```python
from build123d import *

# Parameters (mm, degrees)
SKETCH6_R               = 10
BOSS_EXTRUDE4_DEPTH     = 2.5
SKETCH7_R               = 6
BOSS_EXTRUDE5_DEPTH     = 6.4
SKETCH8_R               = 6
BOSS_EXTRUDE6_DEPTH     = 6.4
CUT_EXTRUDE1_DEPTH      = 7.4
CUT_EXTRUDE1_DEPTH_BACK = 12.4
FILLET1_R               = 0.5


with BuildPart() as part:
    # Sketch6 → Boss-Extrude4 (new body, symmetric)
    with BuildSketch(Plane.XY):
        Circle(SKETCH6_R)
    extrude(amount=BOSS_EXTRUDE4_DEPTH, both=True)

    # Sketch7 → Boss-Extrude5 (add)
    with BuildSketch(Plane.XY.offset(2.5)):
        with Locations((0, 1)):
            Circle(SKETCH7_R)
    extrude(amount=BOSS_EXTRUDE5_DEPTH)

    # Sketch8 → Boss-Extrude6 (add)
    with BuildSketch(Plane(origin=(0, 0, -2.5), x_dir=(-1, 0, 0), z_dir=(0, 0, -1))):
        with Locations((0, -1)):
            Circle(SKETCH8_R)
    extrude(amount=BOSS_EXTRUDE6_DEPTH)

    # Sketch11 → Cut-Extrude1 (cut, two sides)
    with BuildSketch(Plane.XY.offset(2.5)) as cut_extrude1_sk:
        with BuildLine():
            Line((-1.774823935, -2.9), (1.774823935, -2.9))
            ThreePointArc((1.774823935, -2.9), (3.4, 0), (1.774823935, 2.9))
            Line((1.774823935, 2.9), (-1.774823935, 2.9))
            ThreePointArc((-1.774823935, 2.9), (-3.4, 0), (-1.774823935, -2.9))
        make_face()
    extrude(amount=CUT_EXTRUDE1_DEPTH, mode=Mode.SUBTRACT)
    extrude(cut_extrude1_sk.sketch, amount=-CUT_EXTRUDE1_DEPTH_BACK, mode=Mode.SUBTRACT)

    # Fillet1
    fillet1_edges = [part.edges().sort_by_distance(p)[0] for p in [
        (6, -1, -2.5),
        (-6, 1, 2.5),
    ]]
    fillet(fillet1_edges, radius=FILLET1_R)


solid = part.part
```
CAD build for the part. Positions are in the model's coordinates, mm. A direction names the side the tool comes from. Give positions to 0.01 mm unless a question says otherwise; leave off trailing zeros. Order: outer loops, then holes, each group sorted by start corner. A loop starts at its lowest first (then second) coordinate and runs counter-clockwise, first axis right, second up. Notation, with made-up numbers: M 89.25,88.25 L 126.25,88.25 A32 ccw 126.25,116.25 Z; hole C -13,3 d5. An arc over 180 degrees is marked long. Put each result on its own line as item: value. Start each with the question number.
(1) Drill centre lines: line 1 along Y through (x, z) = (1.75, 6.5); line 2 along X through (y, z) = (-0.5, -0.5); line 3 along Y through (x, z) = (-1.5, 2.25). Where is each one in solid material? Low to high.
(2) Which spindle directions (+Z, -Z, +X, -X, +Y, -Y) get a long thin tool onto all of the face, cutting with end or side? Do faces 4 (the flat face through (4, 5, -2.5)), 5 (the flat face through (0, 2.9, 0)), 6 (the cylindrical face through (-6, 1, 6)). Say none if no direction does.
(3) Mould opens along Y. For faces 1 (the flat face through (0, -4, -8.9)), 2 (the cylindrical face through (4.76, -4.65, -5.91)), 3 (the cylindrical face through (-3.4, 0, 0.1)) say: +Y half, -Y half, draft (parallel to the pull), parting line (faces both ways), or undercut.
(4) Flat gauge pins, fed straight in: pin 1 Ø5 at (x, z) = (4.5, -6) entering from +Y; pin 2 Ø8 at (y, z) = (-8, 0.5) entering from +X; pin 3 Ø1.5 at (y, z) = (-3.5, -3) entering from +X. Where does each tip first touch, or does it go through?
(5) Saw through at A-A, the plane x = 0. Write the cut outline in (y, z).
(6) Saw through at B-B, the plane z = 5.75. Write the cut outline in (x, y), then the cut area to 3 significant figures.
(7) Saw through at D-D, the plane y = -8.25. Write the cut outline in (x, z), then the cut area to 3 significant figures.
(8) Saw through at C-C, the plane x = 8. Write the cut outline in (y, z).
Check result:
1. line 1: y = -4.74 to -2.9, 2.9 to 6.74
1. line 2: x = -9.99 to -3.36, 3.36 to 9.99
1. line 3: y = -9.89 to -2.9, 2.9 to 9.89
2. face 4: -Z
2. face 5: +Z, -Z
2. face 6: +Z
3. face 1: draft
3. face 2: parting line
3. face 3: undercut
4. pin 1: stops at y = 4.66
4. pin 2: stops at x = 9.17
4. pin 3: stops at x = 9.56
5. outline: M -10,-2.5 L -7.5,-2.5 A0.5 cw -7,-3 L -7,-8.9 L -2.9,-8.9 L -2.9,8.9 L -5,8.9 L -5,3 A0.5 cw -5.5,2.5 L -10,2.5 Z; M 2.9,-8.9 L 5,-8.9 L 5,-3 A0.5 cw 5.5,-2.5 L 10,-2.5 L 10,2.5 L 7.5,2.5 A0.5 cw 7,3 L 7,8.9 L 2.9,8.9 Z
6. outline: C 0,1 d12; hole M -1.77,-2.9 L 1.77,-2.9 A3.4 ccw 1.77,2.9 L -1.77,2.9 A3.4 ccw Z
6. area: 79.2 mm2
7. outline: M -5.65,-2.5 L 5.65,-2.5 L 5.65,2.5 L -5.65,2.5 Z
7. area: 56.5 mm2
8. outline: M -6,-2.5 L 6,-2.5 L 6,2.5 L -6,2.5 Z
